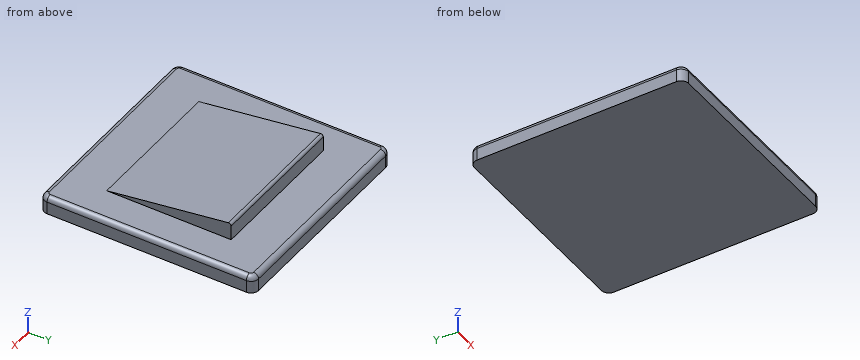
from build123d import *

# Parameters (mm, degrees)
SKETCH_1_W          = 86
SKETCH_1_H          = 86
SKETCH_1_W_2        = 58
SKETCH_1_H_2        = 50
EXTRUDE_1_DEPTH     = 7
SKETCH_1_5_W        = 58
SKETCH_1_5_H        = 50
EXTRUDE_3_DEPTH     = 14
CUT_EXTRUDE_1_DEPTH = 114.030969208
FILLET_1_R          = 3
FILLET_2_R          = 1
FILLET_3_R          = 2


with BuildPart() as part:
    # 草图1 → 凸台-拉伸1 (new body)
    # profile 1 of 2: a face of its own
    with BuildSketch(Plane.XY):
        with Locations((43, 43)):
            Rectangle(SKETCH_1_W, SKETCH_1_H)
        with Locations((43, 43)):
            Rectangle(SKETCH_1_W_2, SKETCH_1_H_2, mode=Mode.SUBTRACT)
    # profile 2 of 2: a face of its own
    with BuildSketch(Plane.XY):
        with Locations((43, 43)):
            Rectangle(SKETCH_1_W_2, SKETCH_1_H_2)
    extrude(amount=EXTRUDE_1_DEPTH)

    # 草图1<5> → 凸台-拉伸3 (add)
    with BuildSketch(Plane.XY):
        with Locations((43, 43)):
            Rectangle(SKETCH_1_5_W, SKETCH_1_5_H)
    extrude(amount=EXTRUDE_3_DEPTH)

    # 草图2 → 切除-拉伸1 (cut, through all)
    with BuildSketch(Plane.ZY.offset(-14)):
        Polygon((14, 68), (7, 18), (14, 18), align=None)
    extrude(amount=-CUT_EXTRUDE_1_DEPTH, mode=Mode.SUBTRACT)

    # 圆角1
    fillet_1_edges = [part.edges().sort_by_distance(p)[0] for p in [
        (0, 0, 3.5),
        (0, 86, 3.5),
        (86, 86, 3.5),
        (86, 0, 3.5),
    ]]
    fillet(fillet_1_edges, radius=FILLET_1_R)

    # 圆角2
    fillet_2_edges = [part.edges().sort_by_distance(p)[0] for p in [
        (43, 68, 14),
    ]]
    fillet(fillet_2_edges, radius=FILLET_2_R)

    # 圆角3
    # the kernel refuses this fillet: 2 mm, written as the material it takes off along each edge
    with BuildSketch(Plane(origin=(83, 86, 7), x_dir=(0, -1, 0), z_dir=(-1, 0, 0)), Plane(origin=(3, 0, 7), x_dir=(0, 1, 0), z_dir=(1, 0, 0)), Plane(origin=(0, 83, 7), x_dir=(1, 0, 0), z_dir=(0, -1, 0))) as fillet_3_piece_1:
        with BuildLine():
            CenterArc((FILLET_3_R, -FILLET_3_R), FILLET_3_R, 90, 90)
            Line((0, -FILLET_3_R), (0, 0))
            Line((0, 0), (FILLET_3_R, 0))
        make_face()
    extrude(amount=80, mode=Mode.SUBTRACT)
    with BuildSketch(Plane(origin=(86, 18, 7), x_dir=(-1, 0, 0), z_dir=(0, 1, 0))) as fillet_3_piece_2:
        with BuildLine():
            CenterArc((FILLET_3_R, -FILLET_3_R), FILLET_3_R, 90, 90)
            Line((0, -FILLET_3_R), (0, 0))
            Line((0, 0), (FILLET_3_R, 0))
        make_face()
    extrude(amount=65, mode=Mode.SUBTRACT)
    with BuildSketch(Plane(origin=(3, 83, 7), x_dir=(-1, 0, 0), z_dir=(0, -1, 0))) as fillet_3_piece_3:
        with BuildLine():
            CenterArc((3 - FILLET_3_R, FILLET_3_R), FILLET_3_R, 270, 90)
            Line((3, FILLET_3_R), (3, 0))
            Line((3, 0), (3 - FILLET_3_R, 0))
        make_face()
    revolve(axis=Axis((3, 83, 7), (0, 0, -1)), revolution_arc=90, mode=Mode.SUBTRACT)
    with BuildSketch(Plane(origin=(3, 3, 7), x_dir=(0, -1, 0), z_dir=(1, 0, 0))) as fillet_3_piece_4:
        with BuildLine():
            CenterArc((3 - FILLET_3_R, FILLET_3_R), FILLET_3_R, 270, 90)
            Line((3, FILLET_3_R), (3, 0))
            Line((3, 0), (3 - FILLET_3_R, 0))
        make_face()
    revolve(axis=Axis((3, 3, 7), (0, 0, -1)), revolution_arc=90, mode=Mode.SUBTRACT)
    with BuildSketch(Plane(origin=(83, 3, 7), x_dir=(0, -1, 0), z_dir=(-1, 0, 0))) as fillet_3_piece_5:
        with BuildLine():
            CenterArc((3 - FILLET_3_R, -FILLET_3_R), FILLET_3_R, 0, 90)
            Line((3, -FILLET_3_R), (3, 0))
            Line((3, 0), (3 - FILLET_3_R, 0))
        make_face()
    revolve(axis=Axis((83, 3, 7), (0, 0, 1)), revolution_arc=90, mode=Mode.SUBTRACT)
    with BuildSketch(Plane(origin=(83, 83, 7), x_dir=(1, 0, 0), z_dir=(0, -1, 0))) as fillet_3_piece_6:
        with BuildLine():
            CenterArc((3 - FILLET_3_R, -FILLET_3_R), FILLET_3_R, 0, 90)
            Line((3, -FILLET_3_R), (3, 0))
            Line((3, 0), (3 - FILLET_3_R, 0))
        make_face()
    revolve(axis=Axis((83, 83, 7), (0, 0, 1)), revolution_arc=90, mode=Mode.SUBTRACT)
    with BuildSketch(Plane(origin=(86, 3, 7), x_dir=(-1, 0, 0), z_dir=(0, 1, 0))) as fillet_3_piece_7:
        with BuildLine():
            CenterArc((FILLET_3_R, -FILLET_3_R), FILLET_3_R, 90, 90)
            Line((0, -FILLET_3_R), (0, 0))
            Line((0, 0), (FILLET_3_R, 0))
        make_face()
    extrude(amount=15, mode=Mode.SUBTRACT)


solid = part.part
Geometry check sheet. Reference: the model listing, model coordinates, mm. Give positions to 0.01 mm unless a question says otherwise; leave off trailing zeros. Write each loop counter-clockwise with the first axis right and the second up, starting at its lowest first coordinate (ties: lowest second). Pieces come first, ordered by that corner, then holes. Notation, with made-up numbers: M 71.5,34.25 L 106.5,34.25 A32 ccw 106.5,62.25 Z; hole C 47,8 d3. An arc over 180 degrees is marked long. Answer as CSV lines item,"result". Start each with the question number.
Q1. Section check D-D, the plane z = 9. Record the cut outline in (x, y), then the cut area to 3 significant figures.
Q2. Section check C-C, the plane y = 15.5. Record the cut outline in (x, z), then the cut area to 3 significant figures.
Q3. Material ranges on L1, parallel to X at y = 57, z = 7.5; L2, parallel to Z at x = 6.5, y = 50; L3, parallel to X at y = 8, z = 6.5, recorded low to high.
Q4. Section check B-B, the plane x = 37. Record the cut outline in (y, z), then the cut area to 3 significant figures.
Q5. Section check A-A, the plane y = 65.5. Record the cut outline in (x, z).
Q6. Go/stop test with flat-tipped pins: pin 1 (2 mm diameter, centred on y = 42, z = 9.5, fed in from +X); pin 2 (4.5 mm diameter, centred on x = 32.5, z = 9.5, fed in from +Y); pin 3 (5 mm diameter, centred on y = 40.5, z = 10, fed in from -X). Record where each tip stops, or that it passes through.
Geometry says:
1,outline,"M 14,32.29 L 72,32.29 L 72,68 L 14,68 Z"
1,area,"2,070 mm^2"
2,outline,"M 0,0 L 86,0 L 86,5 A2 ccw 84,7 L 2,7 A2 ccw 0,5 Z"
2,area,"600 mm^2"
3,L1,"14 to 72"
3,L2,"0 to 7"
3,L3,"0.68 to 85.32"
4,outline,"M 0,0 L 86,0 L 86,5 A2 ccw 84,7 L 68,7 L 68,12.85 A1 ccw 66.86,13.84 L 18,7 L 2,7 A2 ccw 0,5 Z"
4,area,"775 mm^2"
5,outline,"M 0,0 L 86,0 L 86,5 A2 ccw 84,7 L 72,7 L 72,13.65 L 14,13.65 L 14,7 L 2,7 A2 ccw 0,5 Z"
6,pin 1,"x = 72"
6,pin 2,"y = 68"
6,pin 3,"x = 14"
